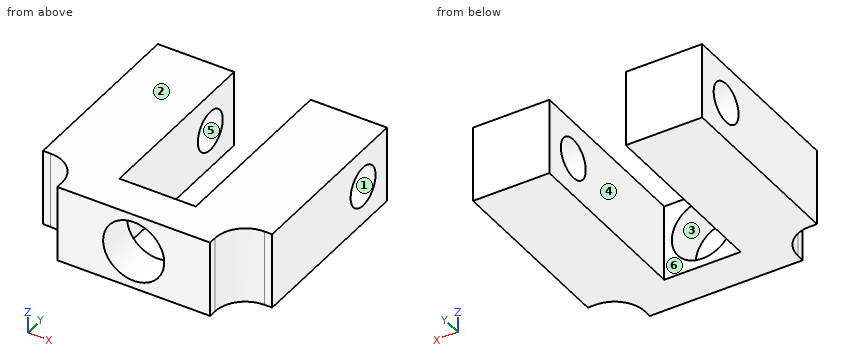
```python
from build123d import *

# Parameters (mm, degrees)
SKETCH1_W           = 12.7
SKETCH1_H           = 6.35
BOSS_EXTRUDE1_DEPTH = 3.175
SKETCH2_W           = 6.35
SKETCH2_H           = 6.35
BOSS_EXTRUDE2_DEPTH = 15.24
FILLET1_R           = 2.54
SKETCH3_R           = 1.651
CUT_EXTRUDE1_DEPTH  = 22.606
SKETCH4_R           = 2.54
CUT_EXTRUDE2_DEPTH  = 22.606


with BuildPart() as part:
    # Sketch1 → Boss-Extrude1 (new body)
    with BuildSketch(Plane(origin=(0, 0, 0), x_dir=(1, 0, 0), z_dir=(0, 1, 0))):
        with Locations((6.35, 3.175)):
            Rectangle(SKETCH1_W, SKETCH1_H)
    extrude(amount=BOSS_EXTRUDE1_DEPTH)

    # Sketch2 → Boss-Extrude2 (add)
    with BuildSketch(Plane(origin=(0, 3.175, 0), x_dir=(1, 0, 0), z_dir=(0, 1, 0))):
        with Locations((0, 3.175)):
            Rectangle(SKETCH2_W, SKETCH2_H)
        with Locations((12.7, 3.175)):
            Rectangle(SKETCH2_W, SKETCH2_H)
    extrude(amount=BOSS_EXTRUDE2_DEPTH)

    # Fillet1
    fillet1_edges = [part.edges().sort_by_distance(p)[0] for p in [
        (12.7, 3.175, -3.175),
        (0, 3.175, -3.175),
    ]]
    fillet(fillet1_edges, radius=FILLET1_R)

    # Sketch3 → Cut-Extrude1 (cut)
    with BuildSketch(Plane.ZY.offset(3.175)):
        with Locations((-3.175, 15.24)):
            Circle(SKETCH3_R)
    extrude(amount=-CUT_EXTRUDE1_DEPTH, mode=Mode.SUBTRACT)

    # Sketch4 → Cut-Extrude2 (cut)
    with BuildSketch(Plane(origin=(0, 3.175, 0), x_dir=(1, 0, 0), z_dir=(0, 1, 0))):
        with Locations(Location((6.35, 3.175, 0), (0, 0, 270))):
            Circle(SKETCH4_R)
    extrude(amount=-CUT_EXTRUDE2_DEPTH, mode=Mode.SUBTRACT)


solid = part.part
```
Source: CAD feature listing. Evaluate the final solid. Frame: model axes, mm. Face numbers are marked on the shaded views. A direction names the side the tool comes from. Give positions to 0.01 mm unless a question says otherwise; leave off trailing zeros. Loops run counter-clockwise (first coordinate to the right, second up) from the corner with the lowest first, then second, coordinate; pieces in that order, holes last. Notation, with made-up numbers: M 22.25,40 L 53.25,40 A13 ccw 53.25,46 Z; hole C 10,77.25 d8. An arc over 180 degrees is marked long. Put each result on its own line as item: value.
Q1. Section B-B (x = 6.35). Return the cut outline in (y, z) (3 decimals).
Response values:
outline: M 0,-6.35 L 3.175,-6.35 L 3.175,-5.715 L 0,-5.715 Z; M 0,-0.635 L 3.175,-0.635 L 3.175,0 L 0,0 Z
Q2. Reachability of the marked faces 5 and 6 from +Z, -Z, +X, -X, +Y, -Y: full face, straight path, thin tool, end or side. Return the list, or none.
Response values:
face 5: +X, -X
face 6: +Z, -Z, +Y
Q3. Section A-A (y = 15.24). Return the cut outline in (x, z) (3 decimals), and give its area (3 significant figures).
Response values:
outline: M -3.175,-6.35 L 3.175,-6.35 L 3.175,-4.826 L -3.175,-4.826 Z; M -3.175,-1.524 L 3.175,-1.524 L 3.175,0 L -3.175,0 Z; M 9.525,-6.35 L 15.875,-6.35 L 15.875,-4.826 L 9.525,-4.826 Z; M 9.525,-1.524 L 15.875,-1.524 L 15.875,0 L 9.525,0 Z
area: 38.7 mm²
Q4. Section D-D (y = 4.75). Return the cut outline in (x, z) (3 decimals).
Response values:
outline: M -3.175,-6.35 L 3.175,-6.35 L 3.175,0 L -3.175,0 Z; M 9.525,-6.35 L 15.875,-6.35 L 15.875,0 L 9.525,0 Z
Q5. Mould query, pull axis Z, two halves, no side actions, for the marked faces 1, 2, 3 and 4. Classes: released by +Z, released by -Z, zero draft, split by the parting line, or undercut.
Response values:
face 1: undercut
face 2: released by +Z
face 3: undercut
face 4: zero draft
Q6. Section C-C (z = -2.5). Return the cut outline in (x, y) (3 decimals).
Response values:
outline: M -3.175,3.175 L -2.54,3.175 A2.54 cw 0,0.635 L 0,0 L 3.901,0 L 3.901,3.175 L 3.175,3.175 L 3.175,13.733 L -3.175,13.733 Z; M -3.175,16.747 L 3.175,16.747 L 3.175,18.415 L -3.175,18.415 Z; M 8.799,0 L 12.7,0 L 12.7,0.635 A2.54 cw 15.24,3.175 L 15.875,3.175 L 15.875,13.733 L 9.525,13.733 L 9.525,3.175 L 8.799,3.175 Z; M 9.525,16.747 L 15.875,16.747 L 15.875,18.415 L 9.525,18.415 Z
Q7. Pin query (flat end, axial travel): P1, Ø5, axis at x = 0.5, y = 12.5, coming from the +Z side; P2, Ø0.5, axis at y = 0, z = -3.5, coming from the +X side; P3, Ø1.5, axis at x = 8.5, z = -5.5, coming from the +Y side (3 decimals); P4, Ø2.5, axis at y = 15.24, z = -3.175, coming from the -X side. Return the tip coordinate at first contact, or that it passes through.
Response values:
P1: stops at z = 0
P2: stops at x = 12.7
P3: stops at y = 3.175
P4: passes through
Q8. Line query: probe 1 along X at (y, z) = (4.75, -6) (3 decimals); probe 2 along Y at (x, z) = (12.5, -2.25) (3 decimals); probe 3 along Y at (x, z) = (0.75, -3) (3 decimals). Output: solid intervals per line, ascending. Write a range as [from, to].
Response values:
probe 1: x = [-3.175, 3.175], [9.525, 15.875]
probe 2: y = [0, 13.872], [16.608, 18.415]
probe 3: y = [0, 13.598], [16.882, 18.415]
